Part print with two shaded views. Sizes in mm from the minimum x, y, z corner. Round coordinates to 2 decimals unless told otherwise and drop trailing zeros. Write each loop counter-clockwise with the first axis right and the second up, starting at its lowest first coordinate (ties: lowest second). Pieces come first, ordered by that corner, then holes. Notation, with made-up numbers: (35, -35) - (50, -35) arc R18 cw to (50, -18) - close; hole circle Ø9 at (6.25, 5.5). An arc over 180 degrees is marked (long way). Answer as a JSON object with one key per item and string values. Group by question number.
Item 1: Slice it at D-D, the plane y = 64. List the corners of the cut face in (x, z), then the cut area to 3 significant figures.
Item 2: Slice it at B-B, the plane z = 75. List the corners of the cut face in (x, y), then the cut area to 3 significant figures.
Item 3: Probe line 1 (Y direction, x = 55.25, z = 88.4); line 2 (X direction, y = 84.45, z = 66.25); line 3 (Y direction, x = 81, z = 44.5). List the from-to ranges inside material, lowest first. Write a range as from..to.
Item 4: Two-plate mould, pull along X, no slides. Class the marked faces 1, 2 and 3: +X half, -X half, draft (parallel to the pull), parting line (faces both ways), or undercut.
Item 5: Flat gauge pins, fed straight in: pin 1 (12 mm diameter, centred on x = 64, y = 71, fed in from -Z); pin 2 (6 mm diameter, centred on y = 77.5, z = 40.5, fed in from +X); pin 3 (5 mm diameter, centred on y = 67.5, z = 19, fed in from -X). Where does each tip first touch, or does it go through?
Item 6: Slice it at A-A, the plane y = 43. List the corners of the cut face in (x, z), then the cut area to 3 significant figures.
Item 7: Slice it at C-C, the plane x = 27.5. List the corners of the cut face in (y, z), then the cut area to 3 significant figures.
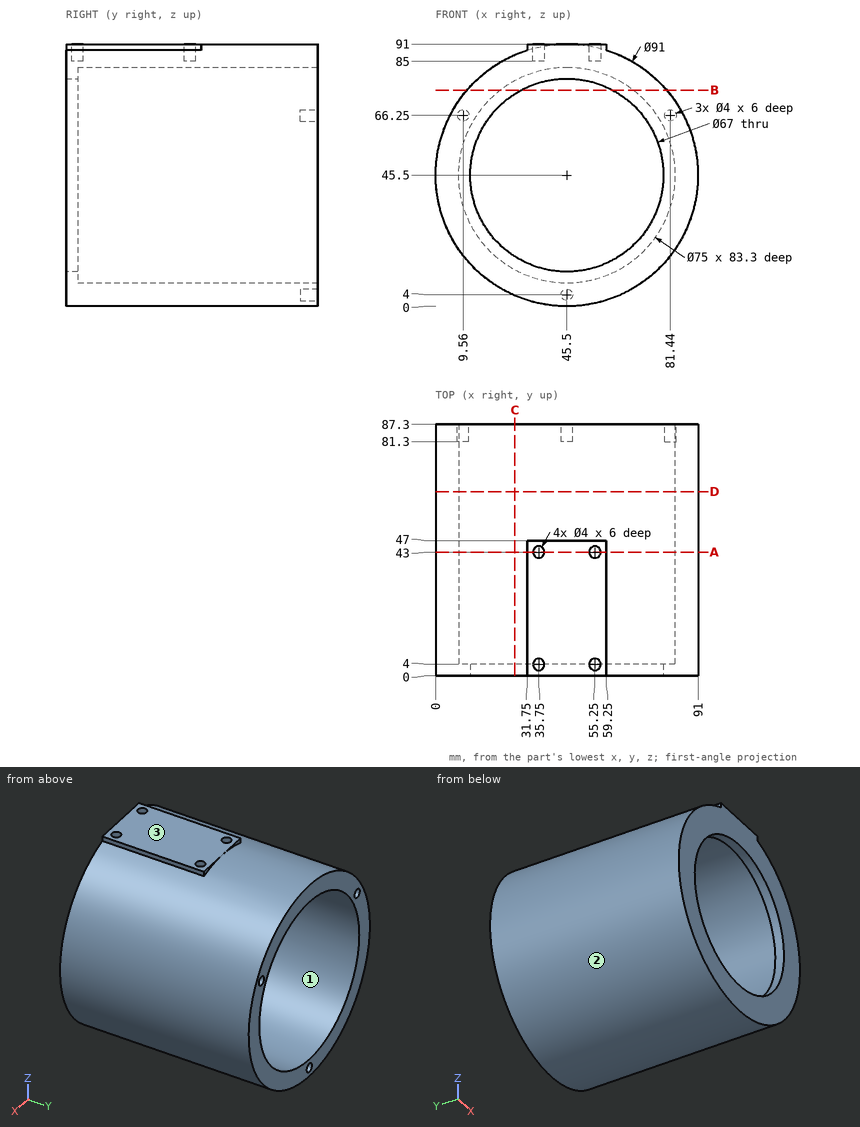
Geometry says:
{
 "1": {"outline": "circle Ø91 at (45.5, 45.5); hole circle Ø75 at (45.5, 45.5)", "area": "2,090 mm^2"},
 "2": {"outline": "(10.86, 0) - (29.63, 0) - (29.63, 4) - (22.35, 4) - (22.35, 87.3) - (10.86, 87.3) - close; (61.37, 0) - (80.14, 0) - (80.14, 87.3) - (68.65, 87.3) - (68.65, 4) - (61.37, 4) - close", "area": "2,060 mm^2"},
 "3": {"line 1": "y = 0..2, 6..41, 45..87.3", "line 2": "x = 5.01..7.56, 11.56..14.26, 76.74..79.44, 83.44..85.99", "line 3": "y = 0..4"},
 "4": {"face 1": "undercut", "face 2": "parting line", "face 3": "draft"},
 "5": {"pin 1": "stops at z = 1.75", "pin 2": "stops at x = 90.96", "pin 3": "stops at x = 6.84"},
 "6": {"outline": "(31.75, 88.87) arc R45.5 ccw (long way) to (59.25, 88.87) - (59.25, 91) - (57.25, 91) - (57.25, 85) - (53.25, 85) - (53.25, 91) - (37.75, 91) - (37.75, 85) - (33.75, 85) - (33.75, 91) - (31.75, 91) - close; hole circle Ø75 at (45.5, 45.5)", "area": "2,060 mm^2"},
 "7": {"outline": "(0, 3.71) - (87.3, 3.71) - (87.3, 12.6) - (4, 12.6) - (4, 17.25) - (0, 17.25) - close; (0, 73.75) - (4, 73.75) - (4, 78.4) - (87.3, 78.4) - (87.3, 87.29) - (0, 87.29) - close", "area": "1,590 mm^2"}
}
